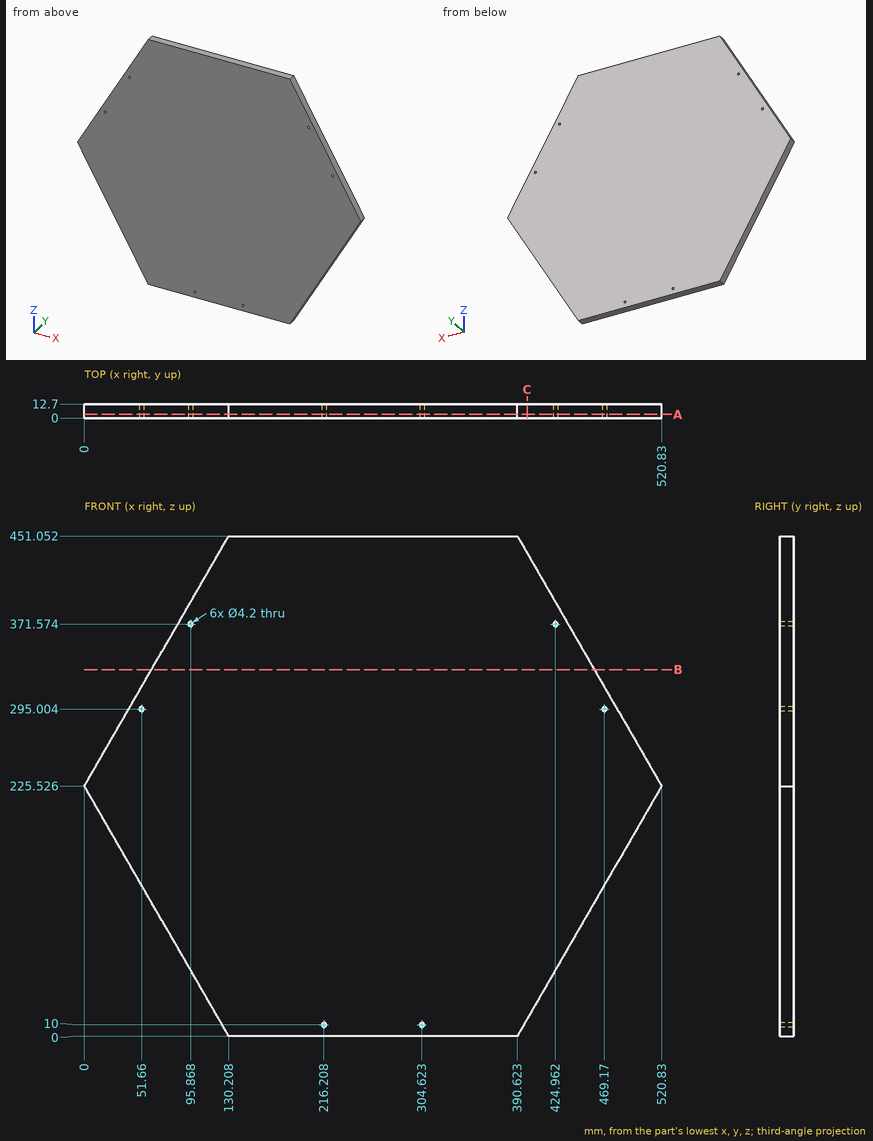
Answer from the drawing. Dimensions are ordinates in mm from the lowest x, y and z of the part. Give positions to 0.01 mm unless a question says otherwise; leave off trailing zeros. Loops run counter-clockwise (first coordinate to the right, second up) from the corner with the lowest first, then second, coordinate; pieces in that order, holes last.
Item 1: Each of these flat-tipped pins is pushed along its axis until it touches: pin 1 Ø4 at (x, y) = (393, 11) entering from -Z (1 decimal); pin 2 Ø2.5 at (x, z) = (95.87, 371.57) entering from +Y; pin 3 Ø1 at (y, z) = (4.5, 182.5) entering from -X; pin 4 Ø1 at (y, z) = (3.5, 379.5) entering from -X. Where does it stop, or does it pass through?
Item 2: The part is cut by section C-C (x = 399.5). Write down the section's boundary in (y, z) (1 decimal).
Item 3: Find the intervals of material crossed by line 1 along X through (y, z) = (9.75, 10) (1 decimal); line 2 along Z through (x, y) = (36, 10.75) (1 decimal); line 3 along X through (y, z) = (11, 73.5), in increasing order.
Item 4: The part is cut by section B-B (z = 330.5). Write down the section's boundary in (x, y).
Item 5: The part is cut by section A-A (y = 3.25). Write down the section's boundary in (x, z) (1 decimal), and give its area (3 significant figures).
Taken from the geometry:
1. pin 1: stops at z = 0.7
1. pin 2: passes through
1. pin 3: stops at x = 24.55
1. pin 4: stops at x = 88.61
2. outline: (0, 15.4) - (12.7, 15.4) - (12.7, 435.7) - (0, 435.7) - close
3. line 1: x = 124.4 to 214.1, 218.3 to 302.5, 306.7 to 396.4
3. line 2: z = 163.2 to 287.9
3. line 3: x = 87.77 to 433.06
4. outline: (60.61, 0) - (460.22, 0) - (460.22, 12.7) - (60.61, 12.7) - close
5. outline: (0, 225.5) - (130.2, 0) - (390.6, 0) - (520.8, 225.5) - (390.6, 451.1) - (130.2, 451.1) - close; hole circle Ø4.2 at (51.7, 295); hole circle Ø4.2 at (95.9, 371.6); hole circle Ø4.2 at (216.2, 10); hole circle Ø4.2 at (304.6, 10); hole circle Ø4.2 at (425, 371.6); hole circle Ø4.2 at (469.2, 295)
5. area: 176,000 mm2
